```python
from build123d import *

# Parameters (mm, degrees)
EXTRUDE_1_DEPTH     = 2
SKETCH_2_R          = 5.6
CUT_EXTRUDE_1_DEPTH = 95.26160406
SKETCH_5_W          = 3
SKETCH_5_H          = 54
EXTRUDE_2_DEPTH     = 10.8
FILLET_1_R          = 2
SKETCH_6_W          = 3
SKETCH_6_H          = 40
CUT_EXTRUDE_3_DEPTH = 6
FILLET_2_R          = 2
FILLET_3_R          = 2


with BuildPart() as part:
    # 草圖1 → 填料-伸長1 (new body)
    with BuildSketch(Plane.XY):
        with BuildLine():
            Line((35.5, 33), (35.5, 29))
            ThreePointArc((35.5, 29), (36.085786438, 27.585786438), (37.5, 27))
            Line((37.5, 27), (85.5, 27))
            ThreePointArc((85.5, 27), (86.914213562, 26.414213562), (87.5, 25))
            Line((87.5, 25), (87.5, -25))
            ThreePointArc((87.5, -25), (86.914213562, -26.414213562), (85.5, -27))
            Line((85.5, -27), (37.5, -27))
            ThreePointArc((37.5, -27), (36.085786438, -27.585786438), (35.5, -29))
            Line((35.5, -29), (35.5, -33))
            ThreePointArc((35.5, -33), (34.914213562, -34.414213562), (33.5, -35))
            Line((33.5, -35), (-33.5, -35))
            ThreePointArc((-33.5, -35), (-34.914213562, -34.414213562), (-35.5, -33))
            Line((-35.5, -33), (-35.5, -29))
            ThreePointArc((-35.5, -29), (-36.085786438, -27.585786438), (-37.5, -27))
            Line((-37.5, -27), (-85.5, -27))
            ThreePointArc((-85.5, -27), (-86.914213562, -26.414213562), (-87.5, -25))
            Line((-87.5, -25), (-87.5, 25))
            ThreePointArc((-87.5, 25), (-86.914213562, 26.414213562), (-85.5, 27))
            Line((-85.5, 27), (-37.5, 27))
            ThreePointArc((-37.5, 27), (-36.085786438, 27.585786438), (-35.5, 29))
            Line((-35.5, 29), (-35.5, 33))
            ThreePointArc((-35.5, 33), (-34.914213562, 34.414213562), (-33.5, 35))
            Line((-33.5, 35), (33.5, 35))
            ThreePointArc((33.5, 35), (34.914213562, 34.414213562), (35.5, 33))
        make_face()
    extrude(amount=EXTRUDE_1_DEPTH)

    # 草圖2 → 除料-伸長1 (cut, through all)
    with BuildSketch(Plane.XY.offset(2)):
        Circle(SKETCH_2_R)
        with BuildLine():
            Line((43.4, -22.5), (43.4, 22.5))
            ThreePointArc((43.4, 22.5), (45, 24.1), (46.6, 22.5))
            Line((46.6, 22.5), (46.6, -22.5))
            ThreePointArc((46.6, -22.5), (45, -24.1), (43.4, -22.5))
        make_face()
        with BuildLine():
            Line((-46.6, -22.5), (-46.6, 22.5))
            ThreePointArc((-46.6, 22.5), (-45, 24.1), (-43.4, 22.5))
            Line((-43.4, 22.5), (-43.4, -22.5))
            ThreePointArc((-43.4, -22.5), (-45, -24.1), (-46.6, -22.5))
        make_face()
        with BuildLine():
            Line((21.5, 28.3), (8.5, 28.3))
            ThreePointArc((8.5, 28.3), (6.8, 30), (8.5, 31.7))
            Line((8.5, 31.7), (21.5, 31.7))
            ThreePointArc((21.5, 31.7), (23.2, 30), (21.5, 28.3))
        make_face()
        with BuildLine():
            Line((-82.6, -22.5), (-82.6, 22.5))
            ThreePointArc((-82.6, 22.5), (-81, 24.1), (-79.4, 22.5))
            Line((-79.4, 22.5), (-79.4, -22.5))
            ThreePointArc((-79.4, -22.5), (-81, -24.1), (-82.6, -22.5))
        make_face()
        with BuildLine():
            Line((79.4, -22.5), (79.4, 22.5))
            ThreePointArc((79.4, 22.5), (81, 24.1), (82.6, 22.5))
            Line((82.6, 22.5), (82.6, -22.5))
            ThreePointArc((82.6, -22.5), (81, -24.1), (79.4, -22.5))
        make_face()
        with BuildLine():
            Line((21.5, 20.8), (8.5, 20.8))
            ThreePointArc((8.5, 20.8), (6.8, 22.5), (8.5, 24.2))
            Line((8.5, 24.2), (21.5, 24.2))
            ThreePointArc((21.5, 24.2), (23.2, 22.5), (21.5, 20.8))
        make_face()
        with BuildLine():
            Line((-21.5, 28.3), (-8.5, 28.3))
            ThreePointArc((-8.5, 28.3), (-6.8, 30), (-8.5, 31.7))
            Line((-8.5, 31.7), (-21.5, 31.7))
            ThreePointArc((-21.5, 31.7), (-23.2, 30), (-21.5, 28.3))
        make_face()
        with BuildLine():
            Line((-21.5, 20.8), (-8.5, 20.8))
            ThreePointArc((-8.5, 20.8), (-6.8, 22.5), (-8.5, 24.2))
            Line((-8.5, 24.2), (-21.5, 24.2))
            ThreePointArc((-21.5, 24.2), (-23.2, 22.5), (-21.5, 20.8))
        make_face()
        with BuildLine():
            Line((21.5, -28.3), (8.5, -28.3))
            ThreePointArc((8.5, -28.3), (6.8, -30), (8.5, -31.7))
            Line((8.5, -31.7), (21.5, -31.7))
            ThreePointArc((21.5, -31.7), (23.2, -30), (21.5, -28.3))
        make_face()
        with BuildLine():
            Line((21.5, -20.8), (8.5, -20.8))
            ThreePointArc((8.5, -20.8), (6.8, -22.5), (8.5, -24.2))
            Line((8.5, -24.2), (21.5, -24.2))
            ThreePointArc((21.5, -24.2), (23.2, -22.5), (21.5, -20.8))
        make_face()
        with BuildLine():
            Line((-21.5, -28.3), (-8.5, -28.3))
            ThreePointArc((-8.5, -28.3), (-6.8, -30), (-8.5, -31.7))
            Line((-8.5, -31.7), (-21.5, -31.7))
            ThreePointArc((-21.5, -31.7), (-23.2, -30), (-21.5, -28.3))
        make_face()
        with BuildLine():
            Line((-21.5, -20.8), (-8.5, -20.8))
            ThreePointArc((-8.5, -20.8), (-6.8, -22.5), (-8.5, -24.2))
            Line((-8.5, -24.2), (-21.5, -24.2))
            ThreePointArc((-21.5, -24.2), (-23.2, -22.5), (-21.5, -20.8))
        make_face()
    extrude(amount=-CUT_EXTRUDE_1_DEPTH, mode=Mode.SUBTRACT)

    # 草圖5 → 填料-伸長2 (add)
    with BuildSketch(Plane.XY.offset(2)):
        with Locations((-53.75, 0)):
            Rectangle(SKETCH_5_W, SKETCH_5_H)
        with Locations((53.75, 0)):
            Rectangle(SKETCH_5_W, SKETCH_5_H)
    extrude(amount=-EXTRUDE_2_DEPTH)

    # 圓角1
    fillet_1_edges = [part.edges().sort_by_distance(p)[0] for p in [
        (55.25, 0, 0),
    ]]
    fillet(fillet_1_edges, radius=FILLET_1_R)

    # 草圖6 → 除料-伸長3 (cut)
    with BuildSketch(Plane(origin=(0, 0, -8.8), x_dir=(-1, 0, 0), z_dir=(0, 0, -1))):
        with Locations((53.75, 0)):
            Rectangle(SKETCH_6_W, SKETCH_6_H)
    extrude(amount=-CUT_EXTRUDE_3_DEPTH, mode=Mode.SUBTRACT)

    # 圓角2
    fillet_2_edges = [part.edges().sort_by_distance(p)[0] for p in [
        (-53.75, -20, -2.8),
        (-53.75, 20, -2.8),
    ]]
    fillet(fillet_2_edges, radius=FILLET_2_R)

    # 圓角3
    fillet_3_edges = [part.edges().sort_by_distance(p)[0] for p in [
        (-55.25, 0, 0),
    ]]
    fillet(fillet_3_edges, radius=FILLET_3_R)


solid = part.part
```
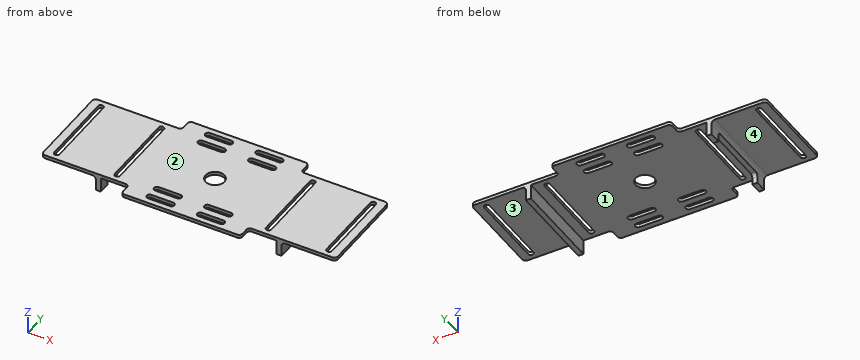
Geometry check sheet. Reference: the model listing, model coordinates, mm. Face numbers are marked on the shaded views. A direction names the side the tool comes from. Give positions to 0.01 mm unless a question says otherwise; leave off trailing zeros. Order: outer loops, then holes, each group sorted by start corner. A loop starts at its lowest first (then second) coordinate and runs counter-clockwise, first axis right, second up.
1. Release check for a two-part mould opening along X. For the marked faces 1 and 2 record: pulls with the +X half, pulls with the -X half, needs draft (parallel to the pull), parting line crosses it, or undercut.
2. Section check A-A, the plane x = -19. Enter the section's corners in (y, z), and give its area (3 significant figures).
3. Access from +Z, -Z, +X, -X, +Y, -Y to the whole of each face (thin tool, end or side, straight path). Record for the marked faces 3 and 4.
4. Section check C-C, the plane x = 45. Enter the section's corners in (y, z), and give its area (3 significant figures).
5. Section check B-B, the plane y = 0. Give the number of separate pieces and of enclosed holes in the cut face, and give its area (3 significant figures).
6. Gauge pin test, flat ends, axial feed: pin 1 Ø0.9 at (x, z) = (-53.5, -7.5) entering from -Y; pin 2 Ø12 at (x, y) = (-13, -19.5) entering from -Z; pin 3 Ø4.5 at (y, z) = (-1.5, -3.5) entering from -X. Record the tip position at first contact, or that the pin passes through.
7. Thickness scan on L1, parallel to X at y = -6, z = 0.5; L2, parallel to Y at x = 0, z = 1.2; L3, parallel to Z at x = -32, y = 25. Record the ranges inside material, lowest first.
Values follow:
1. face 1: undercut
1. face 2: needs draft
2. outline: (-35, 0) - (-31.7, 0) - (-31.7, 2) - (-35, 2) - close; (-28.3, 0) - (-24.2, 0) - (-24.2, 2) - (-28.3, 2) - close; (-20.8, 0) - (20.8, 0) - (20.8, 2) - (-20.8, 2) - close; (24.2, 0) - (28.3, 0) - (28.3, 2) - (24.2, 2) - close; (31.7, 0) - (35, 0) - (35, 2) - (31.7, 2) - close
2. area: 113 mm2
3. face 3: -Z, +X, +Y, -Y
3. face 4: -Z, -X, +Y, -Y
4. outline: (-27, 0) - (-24.1, 0) - (-24.1, 2) - (-27, 2) - close; (24.1, 0) - (27, 0) - (27, 2) - (24.1, 2) - close
4. area: 11.6 mm2
5. separate pieces: 6
5. enclosed holes: 0
5. area: 339 mm2
6. pin 1: stops at y = -27
6. pin 2: stops at z = 0
6. pin 3: stops at x = -55.4
7. L1: x = -87.5 to -82.6, -79.4 to -46.6, -43.4 to 43.4, 46.6 to 79.4, 82.6 to 87.5
7. L2: y = -35 to -5.6, 5.6 to 35
7. L3: z = 0 to 2
